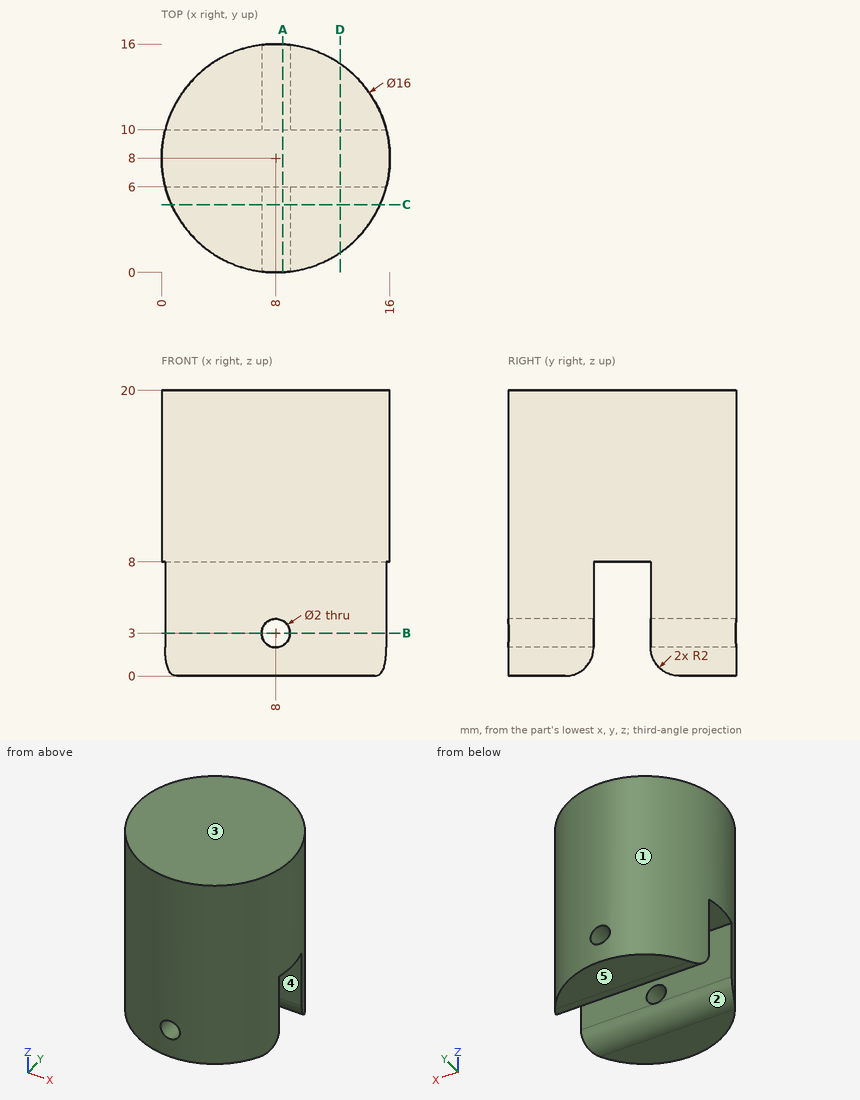
Design review of the part shown in the three views and the two pictorial views. Dimensions are in mm from the part's minimum x, y and z. A direction names the side the tool comes from. Give positions to 0.01 mm unless a question says otherwise; leave off trailing zeros. Write each loop counter-clockwise with the first axis right and the second up, starting at its lowest first coordinate (ties: lowest second). Pieces come first, ordered by that corner, then holes.
(1) Mouldability with a two-part tool opening along Y and no side actions: class the marked faces 1, 2 and 3 as +Y half, -Y half, draft (parallel to the pull), parting line (faces both ways), or undercut.
Checked values:
face 1: parting line
face 2: undercut
face 3: draft
(2) Clearance check with flat-ended pins moving along their axes: pin 1 Ø1.2 at (x, y) = (6.5, 7.5) entering from -Z; pin 2 Ø1.8 at (x, z) = (5.5, 5.5) entering from -Y; pin 3 Ø5 at (y, z) = (3.5, 16.5) entering from +X. State where each tip first meets the part, or that it passes through.
Checked values:
pin 1: stops at z = 8
pin 2: stops at y = 0.16
pin 3: stops at x = 15.75
(3) Tool access review of the marked faces 4 and 5: name each direction out of +Z, -Z, +X, -X, +Y, -Y from which nothing blocks a thin tool from reaching the whole face with its end or side.
Checked values:
face 4: -Z, +X, -X
face 5: -Z, +X, -X, +Y, -Y
(4) Wall thickness on line 1 along Z through (x, y) = (2, 7); line 2 along Z through (x, y) = (8, 11.5); line 3 along Y through (x, z) = (9.75, 4): over which ranges is each line inside the solid? List them lowest first.
Checked values:
line 1: z = 8 to 20
line 2: z = 0.06 to 2, 4 to 20
line 3: y = 0.19 to 6, 10 to 15.81
(5) Add section D-D (x = 12.5). Give the boundary of the cut face in (y, z), and give its area (3 significant figures).
Checked values:
outline: (1.39, 0) - (4, 0) arc R2 ccw to (6, 2) - (6, 8) - (10, 8) - (10, 2) arc R2 ccw to (12, 0) - (14.61, 0) - (14.61, 20) - (1.39, 20) - close
area: 231 mm2
(6) Add section A-A (x = 8.5). Give the boundary of the cut face in (y, z).
Checked values:
outline: (0.02, 0) - (4, 0) arc R2 ccw to (6, 2) - (6, 2.13) - (0.02, 2.13) - close; (0.02, 3.87) - (6, 3.87) - (6, 8) - (10, 8) - (10, 3.87) - (15.98, 3.87) - (15.98, 20) - (0.02, 20) - close; (10, 2) arc R2 ccw to (12, 0) - (15.98, 0) - (15.98, 2.13) - (10, 2.13) - close
(7) Add section B-B (z = 3). Give the boundary of the cut face in (x, y), and give its area (3 significant figures).
Checked values:
outline: (0.25, 6) arc R8 ccw to (7, 0.06) - (7, 6) - close; (0.25, 10) - (7, 10) - (7, 15.94) arc R8 ccw to start; (9, 0.06) arc R8 ccw to (15.75, 6) - (9, 6) - close; (9, 10) - (15.75, 10) arc R8 ccw to (9, 15.94) - close
area: 114 mm2
(8) Add section C-C (y = 4.75). Give the boundary of the cut face in (x, z), and give its area (3 significant figures).
Checked values:
outline: (0.69, 0.15) - (15.31, 0.15) - (15.31, 20) - (0.69, 20) - close; hole circle Ø2 at (8, 3)
area: 287 mm2
